Check sheet for the drawn part. Datum: minimum x, y, z corner. Units: mm. A direction names the side the tool comes from. Coordinates: 2 decimals unless noted, no trailing zeros. Write each loop counter-clockwise with the first axis right and the second up, starting at its lowest first coordinate (ties: lowest second). Pieces come first, ordered by that corner, then holes. Notation, with made-up numbers: (-27, 49) -> (11, 49) arc R22 ccw to (11, 88) -> close; hole circle Ø11 at (33.5, 85.25). An arc over 180 degrees is marked (long way). Answer in a Markdown table with one row per item. Add a question column.
1. Depth check by flat-ended pin: P1, Ø12, axis at y = 16.5, z = 99, coming from the -X side; P2, Ø3, axis at x = 6.5, y = 10.5, coming from the +Z side; P3, Ø12, axis at y = 15, z = 102.5, coming from the +X side; P4, Ø10, axis at x = 31, z = 73.5, coming from the -Y side. Enter the tip coordinate at first touch or a pass-through.
2. Set-up check for the marked faces 1, 2 and 3: record each of +Z, -Z, +X, -X, +Y, -Y from which the full face is reachable in a straight line by a thin tool's end or side.
3. Cross-section at A-A on y = 10.5. Record the cut outline in (x, z), and give its area (3 significant figures).
4. Cross-section at B-B on x = 18. Record the cut outline in (y, z).
5. Scan lines: L1, parallel to Y at x = 20.5, z = 105; L2, parallel to X at y = 1.25, z = 5; L3, parallel to Z at x = 31, y = 6.25. Record each from-to range of solid material in increasing order. Write a range as from..to.
6. Cross-section at C-C on y = 5.5. Record the cut outline in (x, z), and give its area (3 significant figures).
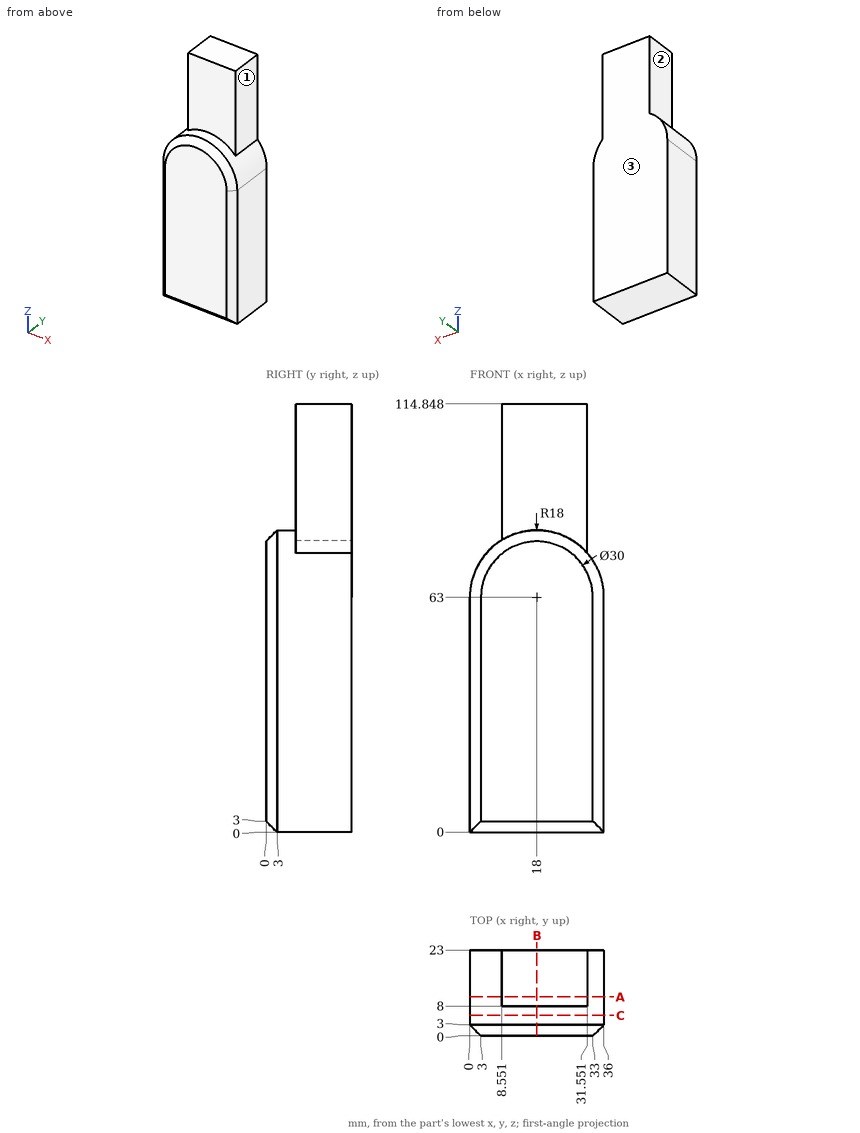
Results found:
| question | item | result |
|---|---|---|
| 1 | P1 | stops at x = 8.55 |
| 1 | P2 | stops at z = 77.97 |
| 1 | P3 | stops at x = 31.55 |
| 1 | P4 | stops at y = 0 |
| 2 | face 1 | +Z, +X, +Y, -Y |
| 2 | face 2 | +Z, -X, +Y, -Y |
| 2 | face 3 | +Z, -Z, +X, -X, +Y |
| 3 | outline | (0, 0) -> (36, 0) -> (36, 63) arc R18 ccw to (31.55, 74.85) -> (31.55, 114.85) -> (8.55, 114.85) -> (8.55, 78.32) arc R18 ccw to (0, 63) -> close |
| 3 | area | 3,590 mm^2 |
| 4 | outline | (0, 3) -> (3, 0) -> (23, 0) -> (23, 114.85) -> (8, 114.85) -> (8, 81) -> (3, 81) -> (0, 78) -> close |
| 5 | L1 | y = 8..23 |
| 5 | L2 | x = 1.75..34.25 |
| 5 | L3 | z = 0..75.45 |
| 6 | outline | (0, 0) -> (36, 0) -> (36, 63) arc R18 ccw to (0, 63) -> close |
| 6 | area | 2,780 mm^2 |
